from build123d import *

# Parameters (mm, degrees)
SKETCH_1_W          = 20
SKETCH_1_H          = 10
SKETCH_1_W_2        = 18
SKETCH_1_H_2        = 8
EXTRUDE_1_DEPTH     = 200
SKETCH_3_R          = 1.6
CUT_EXTRUDE_1_DEPTH = 201.499376558
SKETCH_4_R          = 1.6
CUT_EXTRUDE_2_DEPTH = 202.059692629
SKETCH_5_R          = 1.6
CUT_EXTRUDE_3_DEPTH = 201.499376558
SKETCH_6_R          = 2.1
CUT_EXTRUDE_4_DEPTH = 202.059692629


with BuildPart() as part:
    # 草图1 → 拉伸-薄壁1 (new body)
    with BuildSketch(Plane(origin=(0, 0, 0), x_dir=(1, 0, 0), z_dir=(0, 1, 0))):
        Rectangle(SKETCH_1_W, SKETCH_1_H)
        Rectangle(SKETCH_1_W_2, SKETCH_1_H_2, mode=Mode.SUBTRACT)
    extrude(amount=EXTRUDE_1_DEPTH)

    # 草图3 → 切除-拉伸1 (cut, through all)
    with BuildSketch(Plane.XY.offset(5)):
        with Locations((0, 128)):
            Circle(SKETCH_3_R)
        with Locations(Location((0, 72, 0), (0, 0, 180))):
            Circle(SKETCH_3_R)
    extrude(amount=-CUT_EXTRUDE_1_DEPTH, mode=Mode.SUBTRACT)

    # 草图4 → 切除-拉伸2 (cut, through all)
    with BuildSketch(Plane(origin=(10, 0, 0), x_dir=(0, 0, -1), z_dir=(1, 0, 0))):
        with Locations((0, 109.5)):
            Circle(SKETCH_4_R)
        with Locations((0, 90.5)):
            Circle(SKETCH_4_R)
    extrude(amount=-CUT_EXTRUDE_2_DEPTH, mode=Mode.SUBTRACT)

    # 草图5 → 切除-拉伸3 (cut, through all)
    with BuildSketch(Plane(origin=(0, 0, -5), x_dir=(-1, 0, 0), z_dir=(0, 0, -1))):
        with Locations((-5, 105)):
            Circle(SKETCH_5_R)
        with Locations((-5, 95)):
            Circle(SKETCH_5_R)
        with Locations((5, 95)):
            Circle(SKETCH_5_R)
        with Locations((5, 105)):
            Circle(SKETCH_5_R)
    extrude(amount=-CUT_EXTRUDE_3_DEPTH, mode=Mode.SUBTRACT)

    # 草图6 → 切除-拉伸4 (cut, through all)
    with BuildSketch(Plane(origin=(10, 0, 0), x_dir=(0, 0, -1), z_dir=(1, 0, 0))):
        with Locations((0, 5)):
            Circle(SKETCH_6_R)
        with Locations((0, 15)):
            Circle(SKETCH_6_R)
        with Locations((0, 185)):
            Circle(SKETCH_6_R)
        with Locations((0, 195)):
            Circle(SKETCH_6_R)
    extrude(amount=-CUT_EXTRUDE_4_DEPTH, mode=Mode.SUBTRACT)


solid = part.part
Verification items for the finished model (mm, model axes). A direction names the side the tool comes from. Coordinates: 2 decimals unless noted, no trailing zeros. Order: outer loops, then holes, each group sorted by start corner. A loop starts at its lowest first (then second) coordinate and runs counter-clockwise, first axis right, second up. Notation, with made-up numbers: M 66.5,-8.75 L 74.5,-8.75 A34 ccw 74.5,29.25 Z; hole C 83.25,-4.5 d8. An arc over 180 degrees is marked long. Return JSON: item names as keys, results as strings.
1) Thickness scan on L1, parallel to Y at x = -5, z = 4.5; L2, parallel to X at y = 105, z = 4.4; L3, parallel to Y at x = 0, z = -4.65. Record the ranges inside material, lowest first. Write a range as [from, to].
Answer list:
{"L1": "[0, 93.4], [96.6, 103.4], [106.6, 200]", "L2": "[-10, -6.6], [-3.4, 3.4], [6.6, 10]", "L3": "[0, 70.4], [73.6, 126.4], [129.6, 200]"}
2) Gauge pin test, flat end, axial feed: pin 1 (1.9 mm diameter, centred on x = -5, y = 95, fed in from +Z). Record the tip position at first contact, or that the pin passes through.
Answer list:
{"pin 1": "through"}
3) Release check for a two-part mould opening along Y. For faces 3 (the flat face through (0, 200, 4.4)), 4 (the flat face through (9, 99, 0)), 5 (the cylindrical face through (9.51, 16.77, -1.13)) record: +Y half, -Y half, draft (parallel to the pull), parting line (faces both ways), or undercut.
Answer list:
{"face 3": "+Y half", "face 4": "draft", "face 5": "undercut"}
4) Access from +Z, -Z, +X, -X, +Y, -Y to the whole of each face (thin tool, end or side, straight path). Record for faces 1 (the cylindrical face through (-9.493, 7.082, 0.273)), 2 (the flat face through (-9, 99, 0)).
Answer list:
{"face 1": "+X, -X", "face 2": "+Y, -Y"}
5) Cross-section at B-B, the plane y = 159.5. Record the boundary of the cut face in (x, z).
Answer list:
{"outline": "M -10,-5 L 10,-5 L 10,5 L -10,5 Z; hole M -9,-4 L 9,-4 L 9,4 L -9,4 Z"}
6) Cross-section at A-A, the plane y = 15. Record the boundary of the cut face in (x, z), and give its area (3 significant figures).
Answer list:
{"outline": "M -10,-5 L 10,-5 L 10,-2.1 L 9,-2.1 L 9,-4 L -9,-4 L -9,-2.1 L -10,-2.1 Z; M -10,2.1 L -9,2.1 L -9,4 L 9,4 L 9,2.1 L 10,2.1 L 10,5 L -10,5 Z", "area": "47.6 mm2"}
